The listing builds one solid part. Answer for the finished solid, in the listing's coordinates (mm). Face numbers are marked on the shaded views. Round coordinates to 2 decimals unless told otherwise and drop trailing zeros. Write each loop counter-clockwise with the first axis right and the second up, starting at its lowest first coordinate (ties: lowest second). Pieces come first, ordered by that corner, then holes. Notation, with made-up numbers: M 44,-22 L 79,-22 A33 cw 79,12 Z; hole C 22,69 d9. An arc over 180 degrees is marked long. One line per item, written item: value. Start each with the question number.
(1) Section A-A (x = 2) is taken. Determine the outline of the cut face in (y, z), plus the area to 3 significant figures.
(2) For a pull along X with two mould halves and no side action, classify the marked faces 1, 2 and 3 as released by +X, released by -X, zero draft, split by the parting line, or undercut.
(3) Section B-B (y = -4.25) is taken. Determine the outline of the cut face in (x, z).
(4) Consider probe 1 along Y at (x, z) = (0, 2.25); probe 2 along X at (y, z) = (-3.75, 1.5); probe 3 along Y at (x, z) = (-2, 3.25). Determine where each line is inside the solid, lowest interval first.
(5) Given P1, Ø2, axis at y = -2, z = 5.5, coming from the +X side; P2, Ø1.5, axis at y = 0.5, z = 4.5, coming from the -X side, each flat-ended and moving along its own axis, determine where each tip first touches the part or whether it passes through.
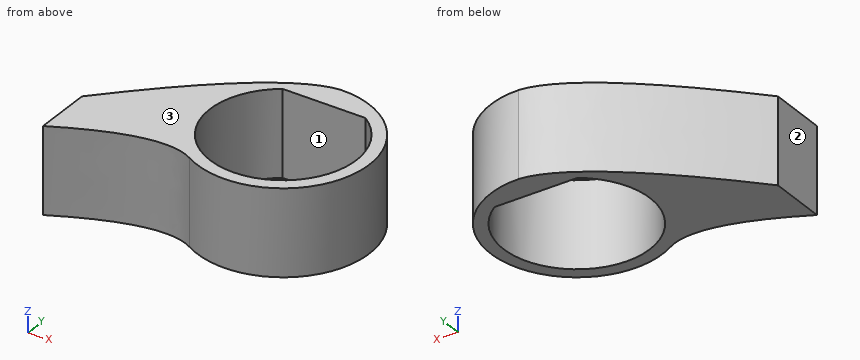
```python
from build123d import *

# Parameters (mm, degrees)
AUFSATZ_LINEAR_AUSTRAGEN1_DEPTH = 6


with BuildPart() as part:
    # Skizze1 → Aufsatz-Linear austragen1 (new body)
    with BuildSketch(Plane.XY):
        with BuildLine():
            Line((-12, -7), (-12, -3))
            add(Edge.make_bspline(
                [(-12, -3), (-3.846414533, 5.771268296), (0, 6)],
                knots=[0, 0, 0, 0.663529029, 0.663529029, 0.663529029], degree=2))
            ThreePointArc((0, 6), (5.795554958, -1.552914271), (-3, -5.196152423))
            add(Edge.make_bspline(
                [(-12, -7), (-5.654241137, -3.663725588), (-3, -5.196152423)],
                knots=[0, 0, 0, 0.361848159, 0.361848159, 0.361848159], degree=2))
        make_face()
        with BuildLine():
            Line((2.893095228, 4.2), (-2.893095228, 4.2))
            ThreePointArc((-2.893095228, 4.2), (0, -5.1), (2.893095228, 4.2))
        make_face(mode=Mode.SUBTRACT)
    extrude(amount=AUFSATZ_LINEAR_AUSTRAGEN1_DEPTH)


solid = part.part
```
Recorded:
1. outline: M -5.66,0 L -4.69,0 L -4.69,6 L -5.66,6 Z; M 4.2,0 L 5.66,0 L 5.66,6 L 4.2,6 Z
1. area: 14.5 mm2
2. face 1: undercut
2. face 2: released by -X
2. face 3: zero draft
3. outline: M -12,0 L -2.82,0 L -2.82,6 L -12,6 Z; M 2.82,0 L 4.24,0 L 4.24,6 L 2.82,6 Z
4. probe 1: y = -6 to -5.1, 4.2 to 6
4. probe 2: x = -12 to -3.46, 3.46 to 4.68
4. probe 3: y = -5.66 to -4.69, 4.2 to 5.44
5. P1: stops at x = 5.92
5. P2: stops at x = -9.34
